```python
from build123d import *

# Parameters (mm, degrees)
BOSS_EXTRUDE1_DEPTH = 6
SKETCH3_W           = 12
SKETCH3_H           = 6
CUT_EXTRUDE1_DEPTH  = 6


with BuildPart() as part:
    # Sketch2 → Boss-Extrude1 (new body)
    with BuildSketch(Plane.XY.offset(-6)):
        Polygon((-152.5, 6), (-138, 6), (-138, 0), (-126, 0), (-126, 6), (-114, 6), (-114, 0), (-102, 0), (-102, 6), (-90, 6), (-90, 0), (-78, 0), (-78, 6), (-66, 6), (-66, 0), (-54, 0), (-54, 6), (-42, 6), (-42, 0), (-30, 0), (-30, 6), (-18, 6), (-18, 0), (-6, 0), (-6, 6), (6, 6), (6, 0), (18, 0), (18, 6), (30, 6), (30, 0), (42, 0), (42, 6), (54, 6), (54, 0), (66, 0), (66, 6), (78, 6), (78, 0), (90, 0), (90, 6), (102, 6), (102, 0), (114, 0), (114, 6), (126, 6), (126, 0), (138, 0), (138, 6), (152.5, 6), (152.5, 0), (158.5, 0), (158.5, -12), (152.5, -12), (152.5, -24), (158.5, -24), (158.5, -36), (152.5, -36), (152.5, -48), (158.5, -48), (158.5, -60), (152.5, -60), (152.5, -66), (-152.5, -66), (-152.5, -60), (-158.5, -60), (-158.5, -48), (-152.5, -48), (-152.5, -36), (-158.5, -36), (-158.5, -24), (-152.5, -24), (-152.5, -12), (-158.5, -12), (-158.5, 0), (-152.5, 0), align=None)
    extrude(amount=BOSS_EXTRUDE1_DEPTH)

    # Sketch3 → Cut-Extrude1 (cut)
    with BuildSketch(Plane.XY):
        with Locations((-132, -63)):
            Rectangle(SKETCH3_W, SKETCH3_H)
        with Locations((-108, -63)):
            Rectangle(SKETCH3_W, SKETCH3_H)
        with Locations((-84, -63)):
            Rectangle(SKETCH3_W, SKETCH3_H)
        with Locations((-60, -63)):
            Rectangle(SKETCH3_W, SKETCH3_H)
        with Locations((-36, -63)):
            Rectangle(SKETCH3_W, SKETCH3_H)
        with Locations((-12, -63)):
            Rectangle(SKETCH3_W, SKETCH3_H)
        with Locations((12, -63)):
            Rectangle(SKETCH3_W, SKETCH3_H)
        with Locations((36, -63)):
            Rectangle(SKETCH3_W, SKETCH3_H)
        with Locations((60, -63)):
            Rectangle(SKETCH3_W, SKETCH3_H)
        with Locations((84, -63)):
            Rectangle(SKETCH3_W, SKETCH3_H)
        with Locations((108, -63)):
            Rectangle(SKETCH3_W, SKETCH3_H)
        with Locations((132, -63)):
            Rectangle(SKETCH3_W, SKETCH3_H)
    extrude(amount=-CUT_EXTRUDE1_DEPTH, mode=Mode.SUBTRACT)


solid = part.part
```
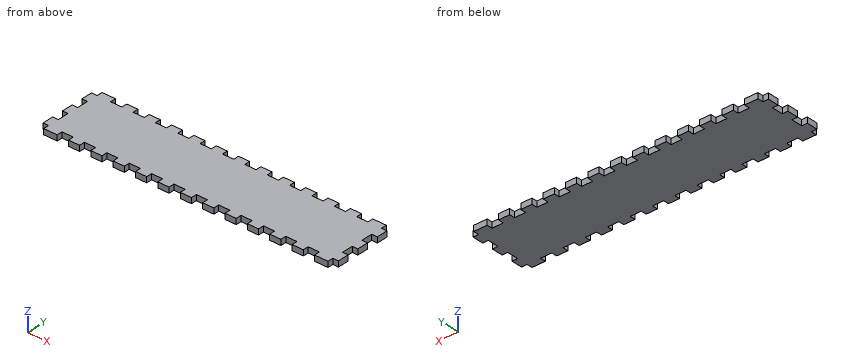
Could you check a few things on this model? Use its own coordinates, in mm. Coordinates: 2 decimals unless noted, no trailing zeros. Loops run counter-clockwise (first coordinate to the right, second up) from the corner with the lowest first, then second, coordinate; pieces in that order, holes last. Notation, with made-up numbers: M 50.5,52.5 L 61.5,52.5 A23 ccw 61.5,76.5 Z; hole C 43,26 d2. An arc over 180 degrees is marked long. Put each result on its own line as item: value. Start each with the question number.
(1) Suppose I cut it at B-B on x = 108. Please give me the cut outline in (y, z).
(2) I need wall thicknesses on line 1 (Y direction, x = -132, z = -3.45); line 2 (X direction, y = -20, z = -2.6). Which ranges of each line are inside material? Lowest first, please. Write a range as from..to.
(3) Will these pins go through, and if not, where does the flat tip stop? P1, Ø3, axis at y = -41, z = -3.5, coming from the -X side; P2, Ø3, axis at x = 36, z = -2, coming from the -Y side; P3, Ø3, axis at y = 4, z = -4, coming from the +X side.
(4) Suppose I cut it at A-A on y = -43. Please give me the cut outline in (x, z), then the cut area to 3 significant figures.
Solutions:
1. outline: M -60,-6 L 0,-6 L 0,0 L -60,0 Z
2. line 1: y = -60..0
2. line 2: x = -152.5..152.5
3. P1: stops at x = -152.5
3. P2: stops at y = -60
3. P3: stops at x = 152.5
4. outline: M -152.5,-6 L 152.5,-6 L 152.5,0 L -152.5,0 Z
4. area: 1,830 mm2
